Verification items for the finished model (mm, model axes). Give positions to 0.01 mm unless a question says otherwise; leave off trailing zeros. Write each loop counter-clockwise with the first axis right and the second up, starting at its lowest first coordinate (ties: lowest second). Pieces come first, ordered by that corner, then holes. Notation, with made-up numbers: (46, -17.75) -> (99, -17.75) arc R16 ccw to (99, 4.25) -> close; hole circle Ø4 at (44.5, -29.75). An arc over 180 degrees is marked (long way). Use CSV: the item, a comma, the result in double quotes. Start each with the question number.
Autodesk Inventor part; units mm, degrees
ref_plane "YZ Plane" through (0, 0, 0) normal (1, 0, 0) x (0, 1, 0)
ref_plane "XZ Plane" through (0, 0, 0) normal (0, 1, 0) x (-1, 0, 0)
ref_plane "XY Plane" through (0, 0, 0) normal (0, 0, 1) x (1, 0, 0)
sketch "Skizze1" plane through (0, 0, 0) normal (0, 1, 0) x (-1, 0, 0)
  line L0 (0, 0) -> (6, 0)
  line L1 (6, 0) -> (6, 10)
  line L2 (6, 10) -> (0, 10)
  line L3 (0, 10) -> (0, 0)
  circle A0 centre (3, 2.9) radius 2.1
  circle A1 centre (3, 7.1) radius 2.1
  dimension "d0" = 6
  dimension "d1" = 10
  dimension "d2" = 4.2
  dimension "d3" = 4.2
  dimension "d4" = 2.9
  dimension "d5" = 2.9
  dimension "d6" = 3
  dimension "d7" = 3
extrude "Extrusion1" add sketch "Skizze1" along normal blind 10
fillet "Rundung1" radius 2 4 edges at (-6, 5, 0) (-6, 5, 10) (0, 5, 10) (0, 5, 0)
equation "\"d7\" = d6"
properties part number "bowden_tube_combiner"
(1) Go/stop test with a flat-tipped pin: pin 1 (2 mm diameter, centred on x = -2, z = 8, fed in from +Y). Record where the tip stops, or that it passes through.
(2) Section check D-D on x = -2.7. Record the cut outline in (y, z), then the cut area to 3 significant figures.
(3) Section check A-A on x = -3.8. Record the cut outline in (y, z).
(4) Thickness scan on line 1 (X direction, y = 8, z = 2.9); line 2 (Z direction, x = -4.7, y = 5.5); line 3 (X direction, y = 3.75, z = 6.25). Record the ranges inside material, lowest first. Write a range as from..to.
(5) Section check C-C on z = 4. Record the cut outline in (x, y), then the cut area to 3 significant figures.
Data:
1,pin 1,"stops at y = 10"
2,outline,"(0, 0) -> (10, 0) -> (10, 0.82) -> (0, 0.82) -> close; (0, 4.98) -> (10, 4.98) -> (10, 5.02) -> (0, 5.02) -> close; (0, 9.18) -> (10, 9.18) -> (10, 10) -> (0, 10) -> close"
2,area,"16.9 mm2"
3,outline,"(0, 0) -> (10, 0) -> (10, 0.96) -> (0, 0.96) -> close; (0, 4.84) -> (10, 4.84) -> (10, 5.16) -> (0, 5.16) -> close; (0, 9.04) -> (10, 9.04) -> (10, 10) -> (0, 10) -> close"
4,line 1,"x = -6..-5.1, -0.9..0"
4,line 2,"z = 0.13..1.67, 4.13..5.87, 8.33..9.87"
4,line 3,"x = -6..-4.92, -1.08..0"
5,outline,"(-6, 0) -> (-4.79, 0) -> (-4.79, 10) -> (-6, 10) -> close; (-1.21, 0) -> (0, 0) -> (0, 10) -> (-1.21, 10) -> close"
5,area,"24.2 mm2"
